Model file for the job. Use its own axes, mm. A direction names the side the tool comes from. Give positions to 0.01 mm unless a question says otherwise; leave off trailing zeros. Write each loop counter-clockwise with the first axis right and the second up, starting at its lowest first coordinate (ties: lowest second). Pieces come first, ordered by that corner, then holes. Notation, with made-up numbers: (7, 4.5) - (37, 4.5) arc R17 ccw to (37, 27.5) - close; hole circle Ø9 at (60, 18.25). An arc over 180 degrees is marked (long way). Use CSV: the item, a comma, the result in double quotes.
Solid Edge part; units mm, degrees
sketch "Sketch1" plane through (0, 0, 0) normal (0, 0, 1) x (1, 0, 0)
  line L0 (34.2, 76) -> (34.2, 0)
  line L1 (34.2, 0) -> (0, 0)
  line L2 (0, 0) -> (0, 76)
  line L3 (0, 76) -> (15, 76)
  line L4 (15, 76) -> (15, 12)
  line L5 (15, 12) -> (19.2, 12)
  line L6 (19.2, 12) -> (19.2, 76)
  line L7 (19.2, 76) -> (34.2, 76)
extrude "Protrusion1" add sketch "Sketch1" along normal blind 4
chamfer "Chaflán_2" distance 4 angle 45 1 edges at (17.1, 12, 4)
(1) Saw through at C-C, the plane z = 3.2. List the corners of the cut face in (x, y), then the cut area to 3 significant figures.
Checked values:
outline,"(0, 0) - (34.2, 0) - (34.2, 76) - (19.2, 76) - (19.2, 8.8) - (15, 8.8) - (15, 76) - (0, 76) - close"
area,"2,320 mm^2"
(2) Wall check: probe 1 along X at (y, z) = (17, 2.8); probe 2 along Y at (x, z) = (18, 1.8); probe 3 along Z at (x, y) = (18.5, 9.5). Give the ranges that are in metal, low to high. Write a range as [from, to].
Checked values:
probe 1,"x = [0, 15], [19.2, 34.2]"
probe 2,"y = [0, 10.2]"
probe 3,"z = [0, 2.5]"
(3) Saw through at A-A, the plane y = 53. List the corners of the cut face in (x, z), then the cut area to 3 significant figures.
Checked values:
outline,"(0, 0) - (15, 0) - (15, 4) - (0, 4) - close; (19.2, 0) - (34.2, 0) - (34.2, 4) - (19.2, 4) - close"
area,"120 mm^2"
(4) 3-axis set-ups, long thin cutter, end or side, ignore diameter. For faces 4 (the face through (17, 0, 2)), 5 (the face through (17, 10, 2)): which of +Z, -Z, +X, -X, +Y, -Y reach the whole face in a straight line?
Checked values:
face 4,"+Z, -Z, +X, -X, -Y"
face 5,"+Z, +Y"
(5) Pull direction X, two halves, no side cores. Call faces 1 (the face through (34.2, 39, 2)), 2 (the face through (15, 42, 2)), 3 (the face through (21, 39, 4)): released by +X, released by -X, zero draft, split by the parting line, or undercut.
Checked values:
face 1,"released by +X"
face 2,"undercut"
face 3,"zero draft"
